from build123d import *

# Parameters (mm, degrees)
F1_DEPTH    = 5
F2_T1_DEPTH = 10
F2_T3_DEPTH = 20
F4_R        = 2
F5_DEPTH    = 10
F6_R        = 2
F7_DEPTH    = 10
F8_R        = 2
F9_DEPTH    = 10


# Not quite as in the source:
# - a fillet or chamfer that OpenCascade refuses, or shapes differently, is made with other operations: its cross-section is extruded or revolved along the edge and cut away or added
# - two fillets or chamfers of one size are made in one step


with BuildPart() as f1:
    # F0 (on Front) → F1 (new body, symmetric)
    with BuildSketch(Plane.XZ):
        with BuildLine():
            Line((-277.5, 60), (-277.5, -60))
            Line((-277.5, -60), (-197.5, -60))
            Line((-197.5, -60), (-197.5, -44.1662961254))
            ThreePointArc((-197.5, -44.1662961254), (-175.6633710032, 7.8544741443), (-127.5852874265, 37.3755985301))
            ThreePointArc((-127.5852874265, 37.3755985301), (-116.7403394644, 39.2599448569), (-105.7578089833, 40))
            Line((-105.7578089833, 40), (105.7578089833, 40))
            ThreePointArc((105.7578089833, 40), (116.7403394644, 39.2599448569), (127.5852874265, 37.3755985301))
            ThreePointArc((127.5852874265, 37.3755985301), (175.6633710032, 7.8544741443), (197.5, -44.1662961254))
            Line((197.5, -44.1662961254), (197.5, -60))
            Line((197.5, -60), (217.5, -60))
            Line((217.5, -60), (217.5, 40))
            Line((217.5, 40), (217.5, 60))
            Line((217.5, 60), (-239.75, 60))
            Line((-239.75, 60), (-239.75, 10))
            ThreePointArc((-239.75, 10), (-247.5, 2.25), (-255.25, 10))
            Line((-255.25, 10), (-255.25, 60))
            Line((-255.25, 60), (-277.5, 60))
        make_face()
    extrude(amount=F1_DEPTH, both=True)

    # F2: fillet of radius 2 on 6 edges, made by hand

    # F2_s2 → F2_t1 (join)
    with BuildSketch(Plane.XZ.offset(-5)):
        with BuildLine():
            ThreePointArc((-197.4924301703, -44.0790595559), (-197.4981066464, -44.1658995935), (-197.5, -44.252904362))
            Line((-197.5, -44.252904362), (-197.5, -44.1662961254))
            ThreePointArc((-197.5, -44.1662961254), (-197.4962254546, -44.1226769409), (-197.4924301703, -44.0790595559))
        make_face()
    extrude(amount=F2_T1_DEPTH)

    # F2_s4 → F2_t3 (cut)
    with BuildSketch(Plane.XZ.offset(-10)):
        with BuildLine():
            ThreePointArc((-255.25, 58), (-255.8357864376, 59.4142135624), (-257.25, 60))
            Line((-257.25, 60), (-255.25, 60))
            Line((-255.25, 60), (-255.25, 58))
        make_face()
        with BuildLine():
            ThreePointArc((-275.5, 60), (-276.9142135624, 59.4142135624), (-277.5, 58))
            Line((-277.5, 58), (-277.5, 60))
            Line((-277.5, 60), (-275.5, 60))
        make_face()
        with BuildLine():
            ThreePointArc((-199.5, -60), (-198.0857864376, -59.4142135624), (-197.5, -58))
            Line((-197.5, -58), (-197.5, -60))
            Line((-197.5, -60), (-199.5, -60))
        make_face()
        with BuildLine():
            ThreePointArc((-237.75, 60), (-239.1642135624, 59.4142135624), (-239.75, 58))
            Line((-239.75, 58), (-239.75, 60))
            Line((-239.75, 60), (-237.75, 60))
        make_face()
        with BuildLine():
            ThreePointArc((217.5, 58), (216.9142135624, 59.4142135624), (215.5, 60))
            Line((215.5, 60), (217.5, 60))
            Line((217.5, 60), (217.5, 58))
        make_face()
    extrude(amount=F2_T3_DEPTH, mode=Mode.SUBTRACT)

    # F4 (on face) → F5 (cut)
    with BuildSketch(Plane.XY.offset(60)):
        with Locations((12.5, 0)):
            Circle(F4_R)
        with Locations((52.5, 0)):
            Circle(F4_R)
    extrude(amount=-F5_DEPTH, mode=Mode.SUBTRACT)

    # F6 (on face) → F7 (cut)
    with BuildSketch(Plane.YZ.offset(217.5)):
        with Locations((0, 46)):
            Circle(F6_R)
    extrude(amount=-F7_DEPTH, mode=Mode.SUBTRACT)

    # F8 (on face) → F9 (cut)
    with BuildSketch(Plane(origin=(-277.5, 0, 0), x_dir=(0, -1, 0), z_dir=(-1, 0, 0))):
        with Locations((0, 50)):
            Circle(F8_R)
    extrude(amount=-F9_DEPTH, mode=Mode.SUBTRACT)


solid = f1.part
Verification items for the finished model (mm, model axes). A direction names the side the tool comes from. Round coordinates to 2 decimals unless told otherwise and drop trailing zeros. Order: outer loops, then holes, each group sorted by start corner. A loop starts at its lowest first (then second) coordinate and runs counter-clockwise, first axis right, second up.
1. Section check A-A on z = 26.5. Record the cut outline in (x, y).
Final values:
outline: (-277.5, -5) - (-255.25, -5) - (-255.25, 5) - (-277.5, 5) - close; (-239.75, -5) - (-153.76, -5) - (-153.76, 5) - (-239.75, 5) - close; (153.76, -5) - (217.5, -5) - (217.5, 5) - (153.76, 5) - close
2. Section check B-B on x = -92.5. Record the cut outline in (y, z), then the cut area to 3 significant figures.
Final values:
outline: (-5, 40) - (5, 40) - (5, 60) - (-5, 60) - close
area: 200 mm2
3. Go/stop test with flat-tipped pins: P1, Ø5, axis at x = -4.5, y = -0.5, coming from the -Z side; P2, Ø1.2, axis at x = 52.5, y = 0.5, coming from the +Z side. Record where each tip stops, or that it passes through.
Final values:
P1: stops at z = 40
P2: stops at z = 50
4. Section check C-C on x = -247.5. Record the cut outline in (y, z).
Final values:
outline: (-5, -60) - (5, -60) - (5, 2.25) - (-5, 2.25) - close
5. Release check for a two-part mould opening along X. For faces 4 (the flat face through (-47.2, 5, 40.3)), 5 (the flat face through (217.5, 0, -2)), 6 (the flat face through (-255.25, 0, 34)), 7 (the cylindrical face through (116.587, -0.07, 39.278)) record: +X half, -X half, draft (parallel to the pull), parting line (faces both ways), or undercut.
Final values:
face 4: draft
face 5: +X half
face 6: undercut
face 7: undercut
6. Access from +Z, -Z, +X, -X, +Y, -Y to the whole of each face (thin tool, end or side, straight path). Record for faces 1 (the flat face through (-239.75, 0, 34)), 2 (the flat face through (-266, 0, 60)), 3 (the flat face through (-1, 0, 40)).
Final values:
face 1: +Z, +Y, -Y
face 2: +Z, +X, -X, +Y, -Y
face 3: -Z, +Y, -Y
7. Thickness scan on L1, parallel to Z at x = 210.75, y = 0; L2, parallel to X at y = 4, z = -50.5; L3, parallel to Y at x = 12.5, z = 56.25. Record the ranges inside material, lowest first.
Final values:
L1: z = -60 to 44, 48 to 60
L2: x = -277.5 to -197.5, 197.5 to 217.5
L3: y = -5 to -2, 2 to 5
